from build123d import *

# Parameters (mm, degrees)
BOSS_EXTRUDE1_DEPTH  = 70
SKETCH2_R            = 1.5
CUT_EXTRUDE1_DEPTH   = 6
LPATTERN1_COUNT      = 4
LPATTERN1_PITCH      = 14
LPATTERN1_COUNT_DIR2 = 2
LPATTERN1_PITCH_DIR2 = 55
SKETCH4_W            = 46.2
SKETCH4_H            = 8
BOSS_EXTRUDE2_DEPTH  = 50
SKETCH5_W            = 46.2
SKETCH5_H            = 8
BOSS_EXTRUDE3_DEPTH  = 50
SKETCH6_W            = 172.2
SKETCH6_H            = 8
BOSS_EXTRUDE4_DEPTH  = 20.1
CIRPATTERN2_COUNT    = 6
SKETCH10_R           = 6.5
CUT_EXTRUDE4_DEPTH   = 10
SKETCH11_R           = 20.2
SKETCH11_R_2         = 1.5
SKETCH11_R_3         = 6.5
BOSS_EXTRUDE6_DEPTH  = 9
SKETCH12_R           = 3
CUT_EXTRUDE5_DEPTH   = 154.13177332


with BuildPart() as part:
    # Sketch1 → Boss-Extrude1 (new body)
    with BuildSketch(Plane.XY):
        Polygon((0, 26.7), (0, 0), (72.2, 0), (72.2, 71.7), (66.2, 71.7), (66.2, 26.7), (55, 26.7), (55, 13.5), (61, 13.5), (61, 18.7), (66.2, 18.7), (66.2, 6), (6, 6), (6, 18.7), (11.2, 18.7), (11.2, 13.5), (17.2, 13.5), (17.2, 26.7), align=None)
    extrude(amount=BOSS_EXTRUDE1_DEPTH)

    # Sketch2 → Cut-Extrude1 (cut)
    with BuildSketch(Plane.ZY.offset(-66.2)):
        with Locations(Location((50.75, 51.5, 0), (0, 0, 270))):
            Circle(SKETCH2_R)
    cut_extrude1 = extrude(amount=-CUT_EXTRUDE1_DEPTH, mode=Mode.SUBTRACT)

    # Sketch3 → Cut-Revolve1 (revolve, cut)
    with BuildSketch(Plane.XZ.offset(-18.7)):
        with BuildLine():
            Line((61.1, 56), (66.1, 56))
            ThreePointArc((66.1, 56), (63.6, 58.5), (61.1, 56))
        make_face()
    cut_revolve1 = revolve(axis=Axis((61.1, 18.7, 56), (1, 0, 0)), mode=Mode.SUBTRACT)

    # LPattern1: Cut-Revolve1 4 × 2
    with Locations(*[(-j * LPATTERN1_PITCH_DIR2, 0, -i * LPATTERN1_PITCH) for i in range(LPATTERN1_COUNT) for j in range(LPATTERN1_COUNT_DIR2) if (i, j) != (0, 0)]):
        add(cut_revolve1, mode=Mode.SUBTRACT)

    # Sketch4 → Boss-Extrude2 (add)
    with BuildSketch(Plane(origin=(72.2, 0, 0), x_dir=(0, 0, -1), z_dir=(1, 0, 0))):
        with Locations((-35, 4)):
            Rectangle(SKETCH4_W, SKETCH4_H)
    extrude(amount=BOSS_EXTRUDE2_DEPTH)

    # Sketch5 → Boss-Extrude3 (add)
    with BuildSketch(Plane.ZY):
        with Locations((35, 4)):
            Rectangle(SKETCH5_W, SKETCH5_H)
    extrude(amount=BOSS_EXTRUDE3_DEPTH)

    # Sketch6 → Boss-Extrude4 (add)
    with BuildSketch(Plane.XZ):
        with Locations((36.1, 54.1)):
            Rectangle(SKETCH6_W, SKETCH6_H)
        with Locations((36.1, 15.9)):
            Rectangle(SKETCH6_W, SKETCH6_H)
    extrude(amount=BOSS_EXTRUDE4_DEPTH)

    # CirPattern2: Cut-Extrude1 ×6 about axis
    cirpattern2_axis = Axis((0, 51.5, 35), (1, 0, 0))
    for i in range(1, CIRPATTERN2_COUNT):
        add(cut_extrude1.rotate(cirpattern2_axis, i * 360 / CIRPATTERN2_COUNT), mode=Mode.SUBTRACT)

    # Sketch10 → Cut-Extrude4 (cut)
    with BuildSketch(Plane.ZY.offset(-66.2)):
        with Locations((35, 44.5)):
            Circle(SKETCH10_R)
    extrude(amount=-CUT_EXTRUDE4_DEPTH, mode=Mode.SUBTRACT)

    # Sketch11 → Boss-Extrude6 (add)
    with BuildSketch(Plane(origin=(72.2, 0, 0), x_dir=(0, 0, -1), z_dir=(1, 0, 0))):
        with Locations(Location((-35, 51.5, 0), (0, 0, 90))):
            Circle(SKETCH11_R)
        with Locations(Location((-42.875, 65.13990011, 0), (0, 0, 210))):
            Circle(SKETCH11_R_2, mode=Mode.SUBTRACT)
        with Locations(Location((-27.125, 65.13990011, 0), (0, 0, 150))):
            Circle(SKETCH11_R_2, mode=Mode.SUBTRACT)
        with Locations(Location((-19.25, 51.5, 0), (0, 0, 90))):
            Circle(SKETCH11_R_2, mode=Mode.SUBTRACT)
        with Locations(Location((-27.125, 37.86009989, 0), (0, 0, 90))):
            Circle(SKETCH11_R_2, mode=Mode.SUBTRACT)
        with Locations(Location((-35, 44.5, 0), (0, 0, 180))):
            Circle(SKETCH11_R_3, mode=Mode.SUBTRACT)
        with Locations(Location((-42.875, 37.86009989, 0), (0, 0, 90))):
            Circle(SKETCH11_R_2, mode=Mode.SUBTRACT)
        with Locations(Location((-50.75, 51.5, 0), (0, 0, 270))):
            Circle(SKETCH11_R_2, mode=Mode.SUBTRACT)
    extrude(amount=BOSS_EXTRUDE6_DEPTH)

    # Sketch12 → Cut-Extrude5 (cut, through all)
    with BuildSketch(Plane(origin=(0, 0, 11.9), x_dir=(-1, 0, 0), z_dir=(0, 0, -1))):
        with Locations(Location((-36.1, -10.1, 0), (0, 0, 90))):
            Circle(SKETCH12_R)
        with Locations(Location((-86.1, -10.1, 0), (0, 0, 90))):
            Circle(SKETCH12_R)
        with Locations(Location((13.9, -10.1, 0), (0, 0, 90))):
            Circle(SKETCH12_R)
    extrude(amount=-CUT_EXTRUDE5_DEPTH, mode=Mode.SUBTRACT)


solid = part.part
Build history of the part. All positions in model axes, mm. A direction names the side the tool comes from. Coordinates: 2 decimals unless noted, no trailing zeros. Write each loop counter-clockwise with the first axis right and the second up, starting at its lowest first coordinate (ties: lowest second). Pieces come first, ordered by that corner, then holes.
(1) Cut at B-B on x = -13.9. List the corners of the cut face in (y, z), and give its area (3 significant figures).
(2) Pin check, flat tips, straight feed: pin 1 Ø4 at (y, z) = (-9, 60.5) entering from -X (3 decimals); pin 2 Ø2 at (x, z) = (32.5, 52.5) entering from +Y; pin 3 Ø4 at (y, z) = (65.14, 27.12) entering from +X; pin 4 Ø2.5 at (x, z) = (62.5, 43) entering from -Y. Stop position of each tip, or through.
(3) Mould opens along Y. For faces 6 (the flat face through (35, 0, 35)), 7 (the flat face through (57, 20, 0)), 8 (the cylindrical face through (-10.926, -10.491, 54.044)) say: pulls with the +Y half, pulls with the -Y half, needs draft (parallel to the pull), parting line crosses it, or undercut.
(4) Cut at C-C on y = 44.5. List the corners of the cut face in (x, z).
(5) Cut at A-A on y = -10.1. State how many separate pieces and enclosed holes the cut face has, and give its area (3 significant figures).
(6) Drill centre lines: line 1 (Y direction, x = 16, z = 5); line 2 (X direction, y = 12.5, z = 59); line 3 (Y direction, x = 74.25, z = 50.75). Where is each one in solid material? Low to high.
(7) Cut at D-D on x = 99. List the corners of the cut face in (y, z), and give its area (3 significant figures).
(8) 3-axis set-ups, long thin cutter, end or side, ignore diameter. For faces 1 (the flat face through (35, -5, 50.1)), 2 (the flat face through (81.2, 51.2, 35.3)), 3 (the flat face through (61, 26.7, 35)), 4 (the flat face through (58, 13.5, 35)), 5 (the flat face through (36, 0, 64)): which of +Z, -Z, +X, -X, +Y, -Y reach the whole face in a straight line?
Working result:
1. outline: (-20.1, 11.9) - (-13.1, 11.9) - (-13.1, 19.9) - (-20.1, 19.9) - close; (-20.1, 50.1) - (-13.1, 50.1) - (-13.1, 58.1) - (-20.1, 58.1) - close; (-7.1, 11.9) - (8, 11.9) - (8, 58.1) - (-7.1, 58.1) - (-7.1, 50.1) - (0, 50.1) - (0, 19.9) - (-7.1, 19.9) - close
1. area: 595 mm2
2. pin 1: passes through
2. pin 2: stops at y = 6
2. pin 3: stops at x = 81.2
2. pin 4: stops at y = 0
3. face 6: pulls with the -Y half
3. face 7: needs draft
3. face 8: undercut
4. outline: (66.2, 0) - (72.2, 0) - (72.2, 16.05) - (81.2, 16.05) - (81.2, 28.5) - (66.2, 28.5) - close; (66.2, 41.5) - (81.2, 41.5) - (81.2, 53.95) - (72.2, 53.95) - (72.2, 70) - (66.2, 70) - close
5. separate pieces: 8
5. enclosed holes: 0
5. area: 2,470 mm2
6. line 1: y = 0 to 6, 13.5 to 26.7
6. line 2: x = 0 to 6, 66.2 to 72.2
6. line 3: y = -20.1 to 8, 38.85 to 50, 53 to 64.15
7. outline: (-20.1, 11.9) - (8, 11.9) - (8, 58.1) - (-20.1, 58.1) - (-20.1, 50.1) - (0, 50.1) - (0, 19.9) - (-20.1, 19.9) - close
7. area: 691 mm2
8. face 1: +X, -X, -Y
8. face 2: +Z, -Z, +X, +Y
8. face 3: +Z, -Z, -X, +Y
8. face 4: +Z, -Z
8. face 5: +Z, +X, -X, -Y
